Geometry check sheet. Reference: the model listing, model coordinates, mm. Round coordinates to 2 decimals unless told otherwise and drop trailing zeros. Loops run counter-clockwise (first coordinate to the right, second up) from the corner with the lowest first, then second, coordinate; pieces in that order, holes last. Notation, with made-up numbers: (66, 56.25) - (92, 56.25) arc R27 ccw to (92, 84.25) - close; hole circle Ø10 at (15, 76). An arc over 180 degrees is marked (long way). Answer in a Markdown table with one row per item. Add a question column.
```python
from build123d import *

# Parameters (mm, degrees)
F0_W     = 33.5071906447
F0_H     = 48.0974167585
F1_DEPTH = 25.4


with BuildPart() as f1:
    # F0 (on Right) → F1 (new body)
    with BuildSketch(Plane.YZ):
        Polygon((31.2226135284, 74.4392722845), (0, 48.0974167585), (33.5071906447, 48.0974167585), align=None)
        Polygon((31.2226135284, 74.4392722845), (33.5071906447, 48.0974167585), (70.0604990125, 74.4392722845), align=None)
        Polygon((33.5071906447, 48.0974167585), (33.5071906447, 0), (70.0604990125, 74.4392722845), align=None)
        with Locations((16.7535953224, 24.0487083793)):
            Rectangle(F0_W, F0_H)
    extrude(amount=F1_DEPTH)


solid = f1.part
```
Q1. Depth check by flat-ended pin: P1, Ø12, axis at x = 4, z = 48, coming from the +Y side; P2, Ø3, axis at x = 3, y = 26, coming from the +Z side; P3, Ø8, axis at x = 7, y = 20.5, coming from the +Z side. Enter the tip coordinate at first touch or a pass-through.
Q2. Scan lines: line 1 (Y direction, x = 6.75, z = 64.5); line 2 (Y direction, x = 4.5, z = 61.5); line 3 (Z direction, x = 3.75, y = 17). Record each from-to range of solid material in increasing order. Write a range as from..to.
Q3. Cross-section at A-A, the plane x = 12. Enter the section's corners in (y, z).
Q4. Cross-section at C-C, the plane z = 53. Enter the section's corners in (x, y).
Q5. Cross-section at B-B, the plane y = 22. Enter the section's corners in (x, z).
Check sheet entries:
| question | item | result |
|---|---|---|
| 1 | P1 | y = 60.02 |
| 1 | P2 | z = 71.3 |
| 1 | P3 | z = 68.77 |
| 2 | line 1 | 19.44..65.18 |
| 2 | line 2 | 15.89..63.71 |
| 2 | line 3 | 0..62.44 |
| 3 | outline | (0, 0) - (33.51, 0) - (70.06, 74.44) - (31.22, 74.44) - (0, 48.1) - close |
| 4 | outline | (0, 5.81) - (25.4, 5.81) - (25.4, 59.53) - (0, 59.53) - close |
| 5 | outline | (0, 0) - (25.4, 0) - (25.4, 66.66) - (0, 66.66) - close |
